Design review of the part shown in the three views and the two pictorial views. Dimensions are in mm from the part's minimum x, y and z. Give positions to 0.01 mm unless a question says otherwise; leave off trailing zeros. Write each loop counter-clockwise with the first axis right and the second up, starting at its lowest first coordinate (ties: lowest second). Pieces come first, ordered by that corner, then holes. Notation, with made-up numbers: (42.25, 42.5) -> (70.25, 42.5) arc R22 ccw to (70.25, 50.5) -> close; hole circle Ø4 at (21, 17.25). An arc over 180 degrees is marked (long way). Use CSV: the item, a comma, the result in double quotes.
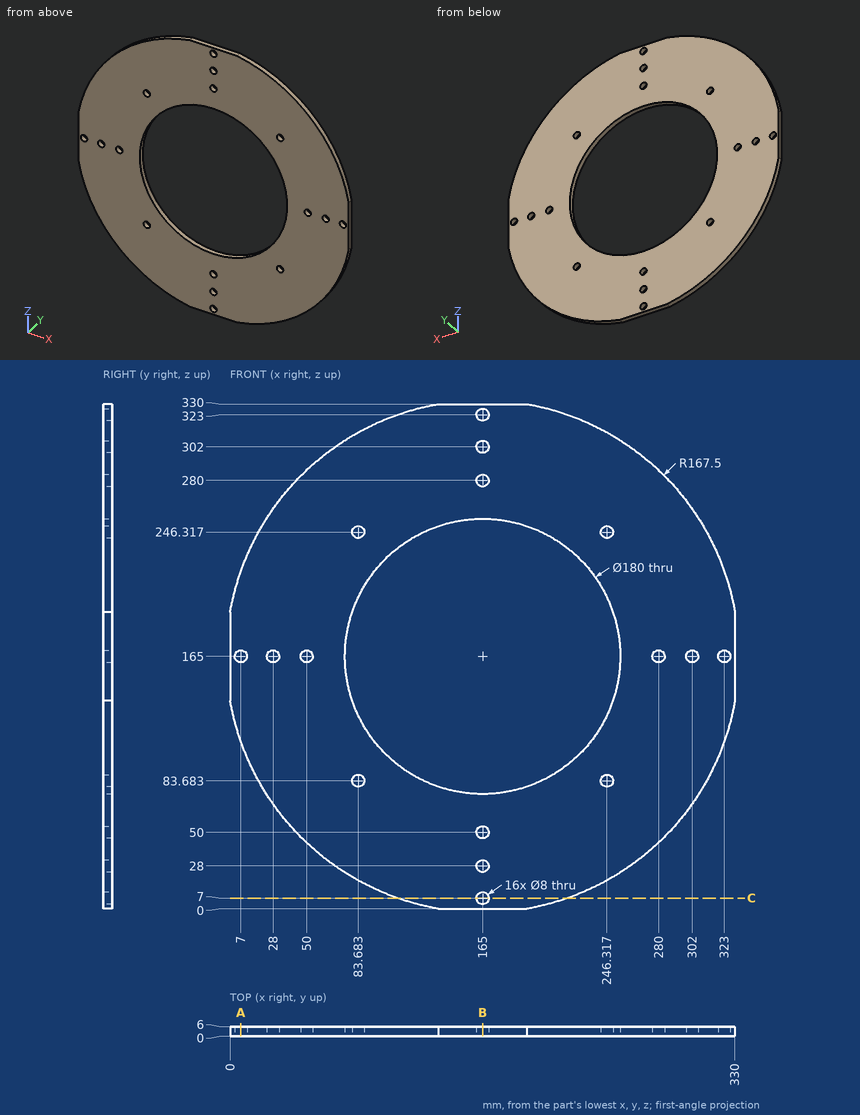
Q1. Consider section A-A (x = 7). Write out the cut boundary in (y, z), then the cut area to 3 significant figures.
Derived:
outline,"(0, 109.39) -> (6, 109.39) -> (6, 161) -> (0, 161) -> close; (0, 169) -> (6, 169) -> (6, 220.61) -> (0, 220.61) -> close"
area,"619 mm2"
Q2. Consider section C-C (z = 7). Write out the cut boundary in (x, y).
Derived:
outline,"(109.39, 0) -> (161, 0) -> (161, 6) -> (109.39, 6) -> close; (169, 0) -> (220.61, 0) -> (220.61, 6) -> (169, 6) -> close"
Q3. Consider section B-B (x = 165). State how many separate pieces and enclosed holes the cut face has, then the cut area to 3 significant figures.
Derived:
separate pieces,"8"
enclosed holes,"0"
area,"612 mm2"
Q4. To check wall thickness, follow probe 1 along Z at (x, y) = (51, 3.5); probe 2 along Z at (x, y) = (206, 0.95) (1 decimal); probe 3 along X at (y, z) = (4.45, 86) (1 decimal). State the ranges of each line that lie inside material, in increasing order.
Derived:
probe 1,"z = 42.28 to 161.13, 168.87 to 287.72"
probe 2,"z = 2.6 to 84.9, 245.1 to 327.4"
probe 3,"x = 17.3 to 80.4, 86.9 to 121.9, 208.1 to 243.1, 249.6 to 312.7"
Q5. Insertion check: pin 1 (7 mm diameter, centred on x = 83.68, z = 246.32, fed in from -Y). The pin has a flat end and moves straight along its axis. Give the tip position at first contact, or say it passes through.
Derived:
pin 1,"passes through"
